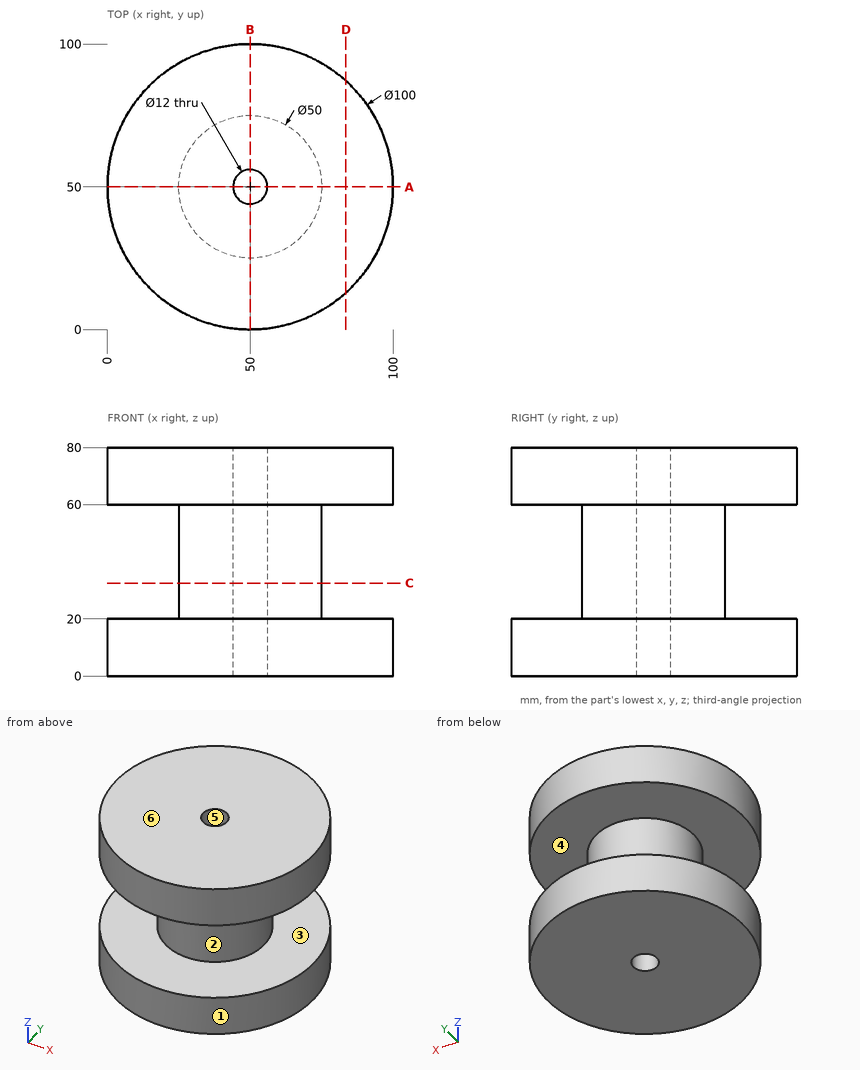
Print and shaded views of the part. All mm, measured from the part's lowest x, y and z. A direction names the side the tool comes from. Give positions to 0.01 mm unless a question says otherwise; leave off trailing zeros. Order: outer loops, then holes, each group sorted by start corner. A loop starts at its lowest first (then second) coordinate and runs counter-clockwise, first axis right, second up. Notation, with made-up numbers: M -17,84 L -3,84 A23 ccw -3,94 Z; hole C -36,67.5 d3. An arc over 180 degrees is marked long. Use one line per item in the form item = value.
Q1. Slice it at C-C, the plane z = 32.5. Write the cut outline in (x, y), and give its area (3 significant figures).
Conclusion:
outline = C 50,50 d50; hole C 50,50 d12
area = 1,850 mm2
Q2. Slice it at A-A, the plane y = 50. Write the cut outline in (x, z), and give its area (3 significant figures).
Conclusion:
outline = M 0,0 L 44,0 L 44,80 L 0,80 L 0,60 L 25,60 L 25,20 L 0,20 Z; M 56,0 L 100,0 L 100,20 L 75,20 L 75,60 L 100,60 L 100,80 L 56,80 Z
area = 5,040 mm2
Q3. Wall check: probe 1 along Y at (x, z) = (50, 17); probe 2 along Z at (x, y) = (45, 5.5); probe 3 along Y at (x, z) = (50, 58.5). Give the ranges that are in metal, low to high.
Conclusion:
probe_1 = 0 to 44, 56 to 100
probe_2 = 0 to 20, 60 to 80
probe_3 = 25 to 44, 56 to 75
Q4. Pin check, flat tips, straight feed: P1, Ø12, axis at y = 20.5, z = 9.5, coming from the +X side; P2, Ø6, axis at y = 30, z = 50, coming from the -X side; P3, Ø4, axis at x = 66, z = 9.5, coming from the -Y side. Stop position of each tip, or through.
Conclusion:
P1 = 94.13
P2 = 31.67
P3 = 2
Q5. Which spindle directions (+Z, -Z, +X, -X, +Y, -Y) get a long thin tool onto all of the face, cutting with end or side? Do the marked faces 1 and 2. Say none if no direction does.
Conclusion:
face_1 = +Z, -Z
face_2 = none
Q6. Slice it at D-D, the plane x = 83.5. Write the cut outline in (y, z), and give its area (3 significant figures).
Conclusion:
outline = M 12.88,0 L 87.12,0 L 87.12,20 L 12.88,20 Z; M 12.88,60 L 87.12,60 L 87.12,80 L 12.88,80 Z
area = 2,970 mm2
Q7. Pull direction Z, two halves, no side cores. Call the marked faces 3, 4, 5 and 6: released by +Z, released by -Z, zero draft, split by the parting line, or undercut.
Conclusion:
face_3 = undercut
face_4 = undercut
face_5 = zero draft
face_6 = released by +Z
